```python
from build123d import *

# Parameters (mm, degrees)
F0_W     = 122
F0_H     = 131
F1_DEPTH = 2
F2_R     = 1
F3_DEPTH = 2.001
F5_W     = 122
F5_H     = 100
F5_W_2   = 120
F5_H_2   = 87
F6_DEPTH = 2
F7_W     = 107
F7_H     = 6.5
F7_W_2   = 1
F7_H_2   = 70
F7_W_3   = 110
F8_DEPTH = 2


with BuildPart() as f1:
    # F0 (on Top) → F1 (new body)
    with BuildSketch(Plane.XY):
        Rectangle(F0_W, F0_H)
    extrude(amount=F1_DEPTH)

    # F2 (on face) → F3 (cut, through all)
    with BuildSketch(Plane.XY.offset(2)):
        with Locations((59, 64)):
            Circle(F2_R)
        with Locations((59, -64)):
            Circle(F2_R)
        with Locations((-59, -64)):
            Circle(F2_R)
        with Locations((-59, 64)):
            Circle(F2_R)
    extrude(amount=-F3_DEPTH, mode=Mode.SUBTRACT)

    # F5 (on face) → F6 (join)
    with BuildSketch(Plane.XY.offset(2)):
        Rectangle(F5_W, F5_H)
        Rectangle(F5_W_2, F5_H_2, mode=Mode.SUBTRACT)
    extrude(amount=F6_DEPTH)

    # F7 (on face) → F8 (cut)
    with BuildSketch(Plane.XY.offset(4)):
        with Locations((0, 46.75)):
            Rectangle(F7_W, F7_H)
        with Locations((60.5, 0)):
            Rectangle(F7_W_2, F7_H_2)
        with Locations((1.5, -46.75)):
            Rectangle(F7_W_3, F7_H)
        with Locations((-60.5, 0)):
            Rectangle(F7_W_2, F7_H_2)
    extrude(amount=-F8_DEPTH, mode=Mode.SUBTRACT)


solid = f1.part
```
Build history of the part. All positions in model axes, mm. Round coordinates to 2 decimals unless told otherwise and drop trailing zeros. Loops run counter-clockwise (first coordinate to the right, second up) from the corner with the lowest first, then second, coordinate; pieces in that order, holes last.
Item 1: Pin check, flat tips, straight feed: P1, Ø1, axis at x = 59.5, z = 3, coming from the -Y side; P2, Ø0.6, axis at x = -56, z = 3, coming from the +Y side; P3, Ø5, axis at x = 27, y = -38.5, coming from the +Z side. Stop position of each tip, or through.
Item 2: Drill centre lines: line 1 along Y through (x, z) = (59, 0.65); line 2 along X through (y, z) = (64, 0.55); line 3 along Z through (x, y) = (-1, -7). Where is each one in solid material? Low to high.
Item 3: Saw through at C-C (y = -17). List the corners of the cut face in (x, z).
Item 4: Saw through at B-B (x = -37). List the corners of the cut face in (y, z).
Item 5: Saw through at A-A (z = 2.85). List the corners of the cut face in (x, y), then the cut area to 4 significant figures.
Worked answers:
1. P1: stops at y = -50
1. P2: stops at y = 50
1. P3: stops at z = 2
2. line 1: y = -65.5 to -65, -63 to 63, 65 to 65.5
2. line 2: x = -61 to -60, -58 to 58, 60 to 61
2. line 3: z = 0 to 2
3. outline: (-61, 0) - (61, 0) - (61, 2) - (-61, 2) - close
4. outline: (-65.5, 0) - (65.5, 0) - (65.5, 2) - (-65.5, 2) - close
5. outline: (-61, -50) - (-53.5, -50) - (-53.5, -43.5) - (-60, -43.5) - (-60, -35) - (-61, -35) - close; (-61, 35) - (-60, 35) - (-60, 43.5) - (-53.5, 43.5) - (-53.5, 50) - (-61, 50) - close; (53.5, 43.5) - (60, 43.5) - (60, 35) - (61, 35) - (61, 50) - (53.5, 50) - close; (56.5, -50) - (61, -50) - (61, -35) - (60, -35) - (60, -43.5) - (56.5, -43.5) - close
5. area: 209.5 mm2
